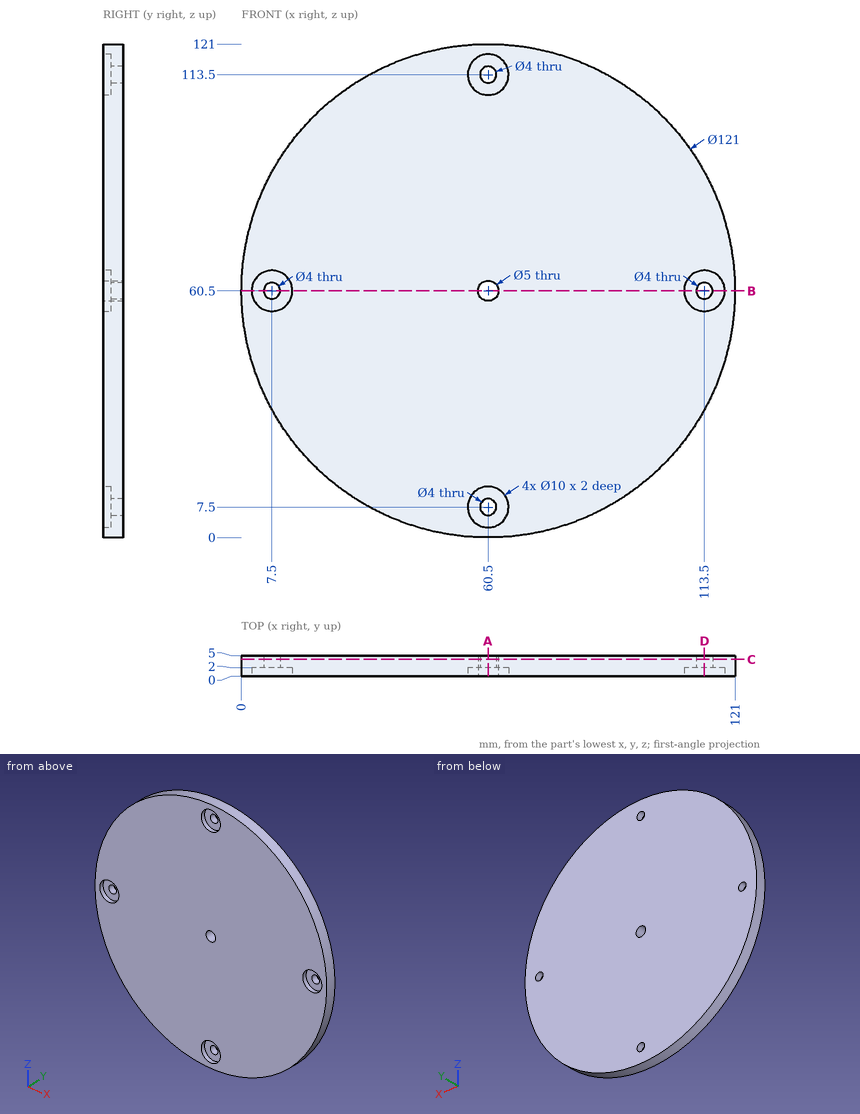
Input: dimensioned drawing with shaded views. Units: mm. Origin: part minimum x, y, z. Give positions to 0.01 mm unless a question says otherwise; leave off trailing zeros. Write each loop counter-clockwise with the first axis right and the second up, starting at its lowest first coordinate (ties: lowest second). Pieces come first, ordered by that corner, then holes. Notation, with made-up numbers: (30, 76.5) - (50, 76.5) arc R16 cw to (50, 80.5) - close; hole circle Ø6 at (-12.75, 69.25). An arc over 180 degrees is marked (long way). One line per item, written item: value. Start each with the question number.
Q1. Section query C-C, the plane y = 4.05. Return the cut outline in (x, z).
Q2. Section query A-A, the plane x = 60.5. Return the cut outline in (y, z).
Q3. Section query D-D, the plane x = 113.5. Return the cut outline in (y, z), then the cut area to 3 significant figures.
Q4. Section query B-B, the plane z = 60.5. Return the cut outline in (x, y), then the cut area to 3 significant figures.
Q5. Material intervals for probe 1 along X at (y, z) = (4.05, 60.5); probe 2 along X at (y, z) = (0.8, 57); probe 3 along X at (y, z) = (1.3, 63.5), sorted ascending. Write a range as from..to.
Q6. First-contact query: pin 1 Ø6 at (x, z) = (113.5, 60.5) entering from -Y; pin 2 Ø8 at (x, z) = (41, 81.5) entering from -Y. Flat tips, straight axial feed; report the tip coordinate or a pass-through.
Answer:
1. outline: circle Ø121 at (60.5, 60.5); hole circle Ø4 at (7.5, 60.5); hole circle Ø5 at (60.5, 60.5); hole circle Ø4 at (60.5, 7.5); hole circle Ø4 at (60.5, 113.5); hole circle Ø4 at (113.5, 60.5)
2. outline: (0, 0) - (5, 0) - (5, 5.5) - (2, 5.5) - (2, 2.5) - (0, 2.5) - close; (0, 12.5) - (2, 12.5) - (2, 9.5) - (5, 9.5) - (5, 58) - (0, 58) - close; (0, 63) - (5, 63) - (5, 111.5) - (2, 111.5) - (2, 108.5) - (0, 108.5) - close; (0, 118.5) - (2, 118.5) - (2, 115.5) - (5, 115.5) - (5, 121) - (0, 121) - close
3. outline: (0, 31.32) - (5, 31.32) - (5, 58.5) - (2, 58.5) - (2, 55.5) - (0, 55.5) - close; (0, 65.5) - (2, 65.5) - (2, 62.5) - (5, 62.5) - (5, 89.68) - (0, 89.68) - close
3. area: 260 mm2
4. outline: (0, 0) - (2.5, 0) - (2.5, 2) - (5.5, 2) - (5.5, 5) - (0, 5) - close; (9.5, 2) - (12.5, 2) - (12.5, 0) - (58, 0) - (58, 5) - (9.5, 5) - close; (63, 0) - (108.5, 0) - (108.5, 2) - (111.5, 2) - (111.5, 5) - (63, 5) - close; (115.5, 2) - (118.5, 2) - (118.5, 0) - (121, 0) - (121, 5) - (115.5, 5) - close
4. area: 516 mm2
5. probe 1: x = 0..5.5, 9.5..58, 63..111.5, 115.5..121
5. probe 2: x = 0.1..3.93, 11.07..109.93, 117.07..120.9
5. probe 3: x = 0.07..3.5, 11.5..109.5, 117.5..120.93
6. pin 1: stops at y = 2
6. pin 2: stops at y = 0
